```python
from build123d import *

# Parameters (mm, degrees)
BOSS_EXTRUDE1_DEPTH      = 6.35
BOSS_EXTRUDE1_DEPTH_BACK = 6.35
BOSS_EXTRUDE2_DEPTH      = 47.625
BOSS_EXTRUDE2_DEPTH_BACK = 66.675
SKETCH3_R                = 3.175
BOSS_EXTRUDE3_DEPTH      = 6.35
SKETCH5_R                = 9.525
BOSS_EXTRUDE4_DEPTH      = 3.175
SKETCH7_R                = 3.175
BOSS_EXTRUDE5_DEPTH      = 25.4
SKETCH8_R                = 6.35
BOSS_EXTRUDE6_DEPTH      = 3.175
SKETCH9_R                = 5.55625
BOSS_EXTRUDE7_DEPTH      = 6.35
FILLET1_R                = 2.54
FILLET1_OF_MIRROR2_R     = 2.54


with BuildPart() as part:
    # Sketch2 → Boss-Extrude1 (new, two sides: drawn at the far end of the back side and taken through both)
    with BuildSketch(Plane(origin=(0, 0, 0), x_dir=(0, 0, -1), z_dir=(1, 0, 0)).offset(-BOSS_EXTRUDE1_DEPTH_BACK)):
        Polygon((4.171210262, -4.874787896), (6.307295287, 1.174980103), (2.136085025, 6.049767999), (-4.171210262, 4.874787896), (-6.307295287, -1.174980103), (-2.136085025, -6.049767999), align=None)
    extrude(amount=BOSS_EXTRUDE1_DEPTH + BOSS_EXTRUDE1_DEPTH_BACK)

    # Sketch3 → Boss-Extrude2 (add, two sides: drawn at the far end of the back side and taken through both)
    with BuildSketch(Plane(origin=(6.35, 0, 0), x_dir=(0, 0, -1), z_dir=(1, 0, 0)).offset(-BOSS_EXTRUDE2_DEPTH_BACK)):
        Circle(SKETCH3_R)
    extrude(amount=BOSS_EXTRUDE2_DEPTH + BOSS_EXTRUDE2_DEPTH_BACK)

    # Sketch4 → Boss-Extrude3 (add)
    with BuildSketch(Plane(origin=(53.975, 0, 0), x_dir=(0, 0, -1), z_dir=(1, 0, 0))):
        Polygon((4.488142835, -4.584662035), (6.214505208, 1.594514693), (1.726362373, 6.179176728), (-4.488142835, 4.584662035), (-6.214505208, -1.594514693), (-1.726362373, -6.179176728), align=None)
    boss_extrude3 = extrude(amount=BOSS_EXTRUDE3_DEPTH)

    # Sketch5 → Boss-Extrude4 (add)
    with BuildSketch(Plane(origin=(60.325, 0, 0), x_dir=(0, 0, -1), z_dir=(1, 0, 0))):
        Circle(SKETCH5_R)
    boss_extrude4 = extrude(amount=BOSS_EXTRUDE4_DEPTH)

    # Mirror1: Boss-Extrude3, Boss-Extrude4 across plane
    add(boss_extrude3.mirror(Plane(origin=(0, 0, 0), x_dir=(0, 0, 1), z_dir=(1, 0, 0))))
    add(boss_extrude4.mirror(Plane(origin=(0, 0, 0), x_dir=(0, 0, 1), z_dir=(1, 0, 0))))

    # Sketch7 → Boss-Extrude5 (add)
    with BuildSketch(Plane(origin=(63.5, 0, 0), x_dir=(0, 0, -1), z_dir=(1, 0, 0))):
        Circle(SKETCH7_R)
    boss_extrude5 = extrude(amount=BOSS_EXTRUDE5_DEPTH)

    # Sketch8 → Boss-Extrude6 (add)
    with BuildSketch(Plane(origin=(88.9, 0, 0), x_dir=(0, 0, -1), z_dir=(1, 0, 0))):
        Circle(SKETCH8_R)
    boss_extrude6 = extrude(amount=BOSS_EXTRUDE6_DEPTH)

    # Sketch9 → Boss-Extrude7 (add)
    with BuildSketch(Plane(origin=(92.075, 0, 0), x_dir=(0, 0, -1), z_dir=(1, 0, 0))):
        Circle(SKETCH9_R)
    boss_extrude7 = extrude(amount=BOSS_EXTRUDE7_DEPTH)

    # Fillet1
    fillet1_edges = [part.edges().sort_by_distance(p)[0] for p in [
        (98.425, 0, 5.55625),
    ]]
    fillet(fillet1_edges, radius=FILLET1_R)

    # Mirror2: Boss-Extrude5, Boss-Extrude6, Boss-Extrude7 across plane
    add(boss_extrude5.mirror(Plane(origin=(0, 0, 0), x_dir=(0, 0, 1), z_dir=(1, 0, 0))))
    add(boss_extrude6.mirror(Plane(origin=(0, 0, 0), x_dir=(0, 0, 1), z_dir=(1, 0, 0))))
    add(boss_extrude7.mirror(Plane(origin=(0, 0, 0), x_dir=(0, 0, 1), z_dir=(1, 0, 0))))

    # Fillet1 of Mirror2
    fillet1_of_mirror2_edges = [part.edges().sort_by_distance(p)[0] for p in [
        (-98.425, 0, 5.55625),
    ]]
    fillet(fillet1_of_mirror2_edges, radius=FILLET1_OF_MIRROR2_R)


solid = part.part
```
Build history of the part. All positions in model axes, mm. A direction names the side the tool comes from. Round coordinates to 2 decimals unless told otherwise and drop trailing zeros. Order: outer loops, then holes, each group sorted by start corner. A loop starts at its lowest first (then second) coordinate and runs counter-clockwise, first axis right, second up. Notation, with made-up numbers: (12, -36) -> (62, -36) arc R18 cw to (62, -22) -> close; hole circle Ø8 at (37.25, -39). An arc over 180 degrees is marked (long way). Answer in a Markdown table with one row per item.
1) Band-saw the part on A-A on x = 49. Give the cut face in (y, z) (3 decimals), and give its area (3 significant figures).
Values:
| item | result |
|---|---|
| outline | circle Ø6.35 at (0, 0) |
| area | 31.7 mm2 |
2) Which spindle directions (+Z, -Z, +X, -X, +Y, -Y) get a long thin tool onto all of the face, cutting with end or side? Do faces 3 (the flat face through (-57.106, -3.855, 4.002)), 4 (the flat face through (-0.089, -1.892, -5.224)), 5 (the flat face through (60.325, -6, 0)), 6 (the flat face through (-0.09, 5.47, 0.97)). Say none if no direction does.
Values:
| item | result |
|---|---|
| face 3 | +Z, -Y |
| face 4 | -Z, -Y |
| face 5 | none |
| face 6 | +Z, +Y |
3) Pin check, flat tips, straight feed: P1, Ø3, axis at x = 42.5, y = 3.5, coming from the -Z side; P2, Ø4, axis at y = 3, z = -2, coming from the +X side (3 decimals); P3, Ø6, axis at x = 13, y = 5, coming from the +Z side; P4, Ø10, axis at y = -7.5, z = 6, coming from the -X side. Stop position of each tip, or through.
Values:
| item | result |
|---|---|
| P1 | z = -2.47 |
| P2 | x = 98.425 |
| P3 | z = 2.47 |
| P4 | x = -97.87 |
4) Wall check: L1, parallel to X at y = 5.5, z = -2.25 (3 decimals); L2, parallel to X at y = 3.75, z = 8 (3 decimals); L3, parallel to X at y = 3.5, z = -4 (3 decimals). Give the ranges that are in metal, low to high.
Values:
| item | result |
|---|---|
| L1 | -92.075 to -88.9, -63.5 to -53.975, -6.35 to 6.35, 53.975 to 63.5, 88.9 to 92.075 |
| L2 | -63.5 to -60.325, 60.325 to 63.5 |
| L3 | -96.965 to -88.9, -63.5 to -53.975, -6.35 to 6.35, 53.975 to 63.5, 88.9 to 96.965 |
5) Mould opens along X. For faces 1 (the flat face through (-60.325, -6, 0)), 2 (the cylindrical face through (61.89, -5.796, 7.559)) say: released by +X, released by -X, zero draft, split by the parting line, or undercut.
Values:
| item | result |
|---|---|
| face 1 | undercut |
| face 2 | zero draft |
